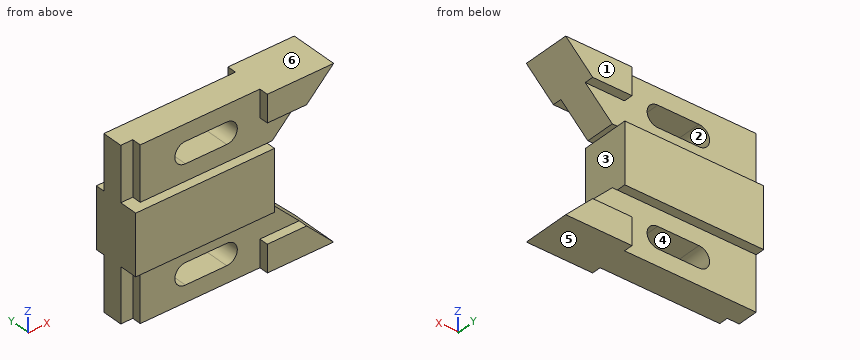
```python
from build123d import *

# Parameters (mm, degrees)
F1_DEPTH      = 12.7
F2_DEPTH      = 7.874
F0_W          = 6.35
F0_H          = 28.575
F3_DEPTH      = 3.048
F3_DEPTH_BACK = 7.874
F4_DEPTH      = 12.7


with BuildPart() as f1:
    # F0 (on Front) → F1 (new body, symmetric)
    with BuildSketch(Plane.XZ):
        Polygon((69.596, 14.2875), (90.3605, 14.2875), (104.648, 28.575), (69.596, 28.575), align=None)
    extrude(amount=F1_DEPTH, both=True)

    # F0 (on Front) → F2 (join, symmetric)
    with BuildSketch(Plane.XZ):
        Polygon((73.406, 0), (76.073, 0), (90.3605, 14.2875), (69.596, 14.2875), (69.596, 28.575), (6.35, 28.575), (6.35, 0), align=None)
        with BuildLine():
            ThreePointArc((52.07, 19.8755), (57.658, 14.2875), (52.07, 8.6995))
            Line((52.07, 8.6995), (30.226, 8.6995))
            ThreePointArc((30.226, 8.6995), (24.638, 14.2875), (30.226, 19.8755))
            Line((30.226, 19.8755), (52.07, 19.8755))
        make_face(mode=Mode.SUBTRACT)
    extrude(amount=F2_DEPTH, both=True)

    # F0 (on Front) → F3 (join, two sides)
    with BuildSketch(Plane.XZ) as f3_sk:
        with Locations((3.175, 14.2875)):
            Rectangle(F0_W, F0_H)
    extrude(amount=F3_DEPTH)
    extrude(f3_sk.sketch, amount=-F3_DEPTH_BACK)

    # F0 (on Front) → F4 (join, symmetric)
    with BuildSketch(Plane.XZ):
        Polygon((73.406, -15.875), (73.406, 0), (6.35, 0), (0, 0), (0, -15.875), align=None)
    extrude(amount=F4_DEPTH, both=True)

    # F5: F1 across face


with BuildPart() as f1_1:
    add(f1.part)
    add(f1.part.mirror(Plane(origin=(36.703, 0, -15.875), x_dir=(1, 0, 0), z_dir=(0, 0, -1))))


solid = f1_1.part
```
Source: CAD feature listing. Evaluate the final solid. Frame: model axes, mm. Face numbers are marked on the shaded views. A direction names the side the tool comes from. Coordinates: 2 decimals unless noted, no trailing zeros. Write each loop counter-clockwise with the first axis right and the second up, starting at its lowest first coordinate (ties: lowest second). Pieces come first, ordered by that corner, then holes. Notation, with made-up numbers: (29, 88) -> (54, 88) arc R24 cw to (54, 117) -> close; hole circle Ø4 at (40.25, 68). An arc over 180 degrees is marked (long way). Return JSON: item names as keys, results as strings. Group by question number.
1) Section query A-A, the plane x = 43. State how many separate pieces and enclosed holes the cut face has, plus the area to 3 significant figures.
2) Contact query for flat-ended pins moving along their axis: P1, Ø2.5, axis at y = -5, z = -42.5, coming from the -X side; P2, Ø4, axis at y = 10.5, z = -49.5, coming from the -X side; P3, Ø2, axis at x = 84.5, z = -41, coming from the +Y side. Output: stop coordinate, or through.
3) Set-up query: the marked faces 1, 2 and 3. Return all of +Z, -Z, +X, -X, +Y, -Y with unobstructed straight access to the full face (end or side cutting, diameter ignored); none if empty.
4) Section query D-D, the plane x = 63.5. Return loops of the section in (y, z) (3 decimals).
5) Ray query, line 1 along Z through (x, y) = (36, -3) (1 decimal); line 2 along X through (y, z) = (11.5, -18.5); line 3 along Z through (x, y) = (57, -5.75) (3 decimals). Return the intervals inside material, ascending.
6) Mould query, pull axis Z, two halves, no side actions, for the marked faces 4, 5 and 6. Classes: +Z half, -Z half, draft (parallel to the pull), parting line (faces both ways), or undercut.
From the geometry:
{
 "1": {"separate pieces": "3", "enclosed holes": "0", "area": "1,350 mm²"},
 "2": {"P1": "x = 6.35", "P2": "x = 69.6", "P3": "y = 7.87"},
 "3": {"face 1": "+Z, -Z, +X, -X, +Y", "face 2": "+Y, -Y", "face 3": "+X, +Y, -Y"},
 "4": {"outline": "(-12.7, -31.75) -> (-7.874, -31.75) -> (-7.874, -60.325) -> (7.874, -60.325) -> (7.874, -31.75) -> (12.7, -31.75) -> (12.7, 0) -> (7.874, 0) -> (7.874, 28.575) -> (-7.874, 28.575) -> (-7.874, 0) -> (-12.7, 0) -> close"},
 "5": {"line 1": "-60.3 to -51.6, -40.4 to 8.7, 19.9 to 28.6", "line 2": "0 to 73.41", "line 3": "-60.325 to -48.668, -43.407 to 11.657, 16.918 to 28.575"},
 "6": {"face 4": "undercut", "face 5": "-Z half", "face 6": "+Z half"}
}
